Input: part model. Units: mm. Frame: model coordinates. A direction names the side the tool comes from. Coordinates: 2 decimals unless noted, no trailing zeros. Write each loop counter-clockwise with the first axis right and the second up, starting at its lowest first coordinate (ties: lowest second). Pieces come first, ordered by that corner, then holes. Notation, with made-up numbers: (26, -11.75) - (47, -11.75) arc R17 cw to (47, 11.25) - close; hole circle Ø1 at (11, 72.25). An arc over 180 degrees is marked (long way). Use a Markdown table: item, result. Add a question column.
Q1. Section query C-C (y = -1.5). Return the cut outline in (x, z).
Q2. Material intervals for probe 1 along Y at (x, z) = (25.4, 7.2); probe 2 along Z at (x, y) = (-19.05, 0.1); probe 3 along Z at (x, y) = (2.5, -11), sorted ascending. Write a range as from..to.
Q3. Section query A-A (x = -25.4). Return the cut outline in (y, z).
Q4. Mould query, pull axis X, two halves, no side actions, for faces 1 (the face through (-17.4, -0.01, -0.68)), 2 (the face through (-1, -9, 6.35)). Classes: released by +X, released by -X, zero draft, split by the parting line, or undercut.
Q5. Section query B-B (z = 0). Return the cut outline in (x, y).
Q6. Pin query (flat end, axial travel): P1, Ø3, axis at x = 6.5, y = -4.5, coming from the -Z side; P2, Ø3, axis at x = -19.05, z = 0, coming from the -Y side; P3, Ø1, axis at y = -2, z = 6, coming from the -X side; P4, Ø7, axis at x = 6, z = -3, coming from the -Y side. Return the tip coordinate at first contact, or that it passes through.
Q7. Set-up query: faces 3 (the face through (-1, -0.794, -1)), 4 (the face through (-1, -16.669, 7)). Return all of +Z, -Z, +X, -X, +Y, -Y with unobstructed straight access to the full face (end or side cutting, diameter ignored); none if empty.
Q8. Section query D-D (z = -3.5). Return the cut outline in (x, y).
from build123d import *

# Parameters (mm, degrees)
F0_W      = 76.2
F0_H      = 15.875
F1_DEPTH  = 0.79375
F2_R      = 1.7859375
F3_DEPTH  = 1.5885
F4_R      = 1.7859375
F5_DEPTH  = 1.5885
F6_W      = 76.2
F6_H      = 1.5875
F7_DEPTH  = 15.875
F8_R      = 1.7859375
F9_DEPTH  = 1.5885
F10_R     = 1.7859375
F11_DEPTH = 1.5885


with BuildPart() as f1:
    # F0 (on Front) → F1 (new body, symmetric)
    with BuildSketch(Plane.XZ):
        Rectangle(F0_W, F0_H)
    extrude(amount=F1_DEPTH, both=True)

    # F2 (on face) → F3 (cut, through all)
    with BuildSketch(Plane.XZ.offset(0.79375)):
        with Locations((-19.05, 0)):
            Circle(F2_R)
    extrude(amount=-F3_DEPTH, mode=Mode.SUBTRACT)

    # F4 (on face) → F5 (cut, through all)
    with BuildSketch(Plane.XZ.offset(0.79375)):
        with Locations((19.05, 0)):
            Circle(F4_R)
    extrude(amount=-F5_DEPTH, mode=Mode.SUBTRACT)

    # F6 (on face) → F7 (join)
    with BuildSketch(Plane.XZ.offset(0.79375)):
        with Locations((0, 7.14375)):
            Rectangle(F6_W, F6_H)
    extrude(amount=F7_DEPTH)

    # F8 (on face) → F9 (cut, through all)
    with BuildSketch(Plane(origin=(0, 0, 6.35), x_dir=(1, 0, 0), z_dir=(0, 0, -1))):
        with Locations((-25.4, 7.14375)):
            Circle(F8_R)
    extrude(amount=-F9_DEPTH, mode=Mode.SUBTRACT)

    # F10 (on face) → F11 (cut, through all)
    with BuildSketch(Plane(origin=(0, 0, 6.35), x_dir=(1, 0, 0), z_dir=(0, 0, -1))):
        with Locations((25.4, 7.14375)):
            Circle(F10_R)
    extrude(amount=-F11_DEPTH, mode=Mode.SUBTRACT)


solid = f1.part
Values follow:
| question | item | result |
|---|---|---|
| 1 | outline | (-38.1, 6.35) - (38.1, 6.35) - (38.1, 7.94) - (-38.1, 7.94) - close |
| 2 | probe 1 | -16.67..-8.93, -5.36..0.79 |
| 2 | probe 2 | -7.94..-1.79, 1.79..7.94 |
| 2 | probe 3 | 6.35..7.94 |
| 3 | outline | (-16.67, 6.35) - (-8.93, 6.35) - (-8.93, 7.94) - (-16.67, 7.94) - close; (-5.36, 6.35) - (-0.79, 6.35) - (-0.79, -7.94) - (0.79, -7.94) - (0.79, 7.94) - (-5.36, 7.94) - close |
| 4 | face 1 | undercut |
| 4 | face 2 | zero draft |
| 5 | outline | (-38.1, -0.79) - (-20.84, -0.79) - (-20.84, 0.79) - (-38.1, 0.79) - close; (-17.26, -0.79) - (17.26, -0.79) - (17.26, 0.79) - (-17.26, 0.79) - close; (20.84, -0.79) - (38.1, -0.79) - (38.1, 0.79) - (20.84, 0.79) - close |
| 6 | P1 | z = 6.35 |
| 6 | P2 | through |
| 6 | P3 | x = -38.1 |
| 6 | P4 | y = -0.79 |
| 7 | face 3 | -Z, +X, -X, -Y |
| 7 | face 4 | +Z, -Z, +X, -X, -Y |
| 8 | outline | (-38.1, -0.79) - (38.1, -0.79) - (38.1, 0.79) - (-38.1, 0.79) - close |
